from build123d import *

# Parameters (mm, degrees)
F0_R     = 25.4
F0_R_2   = 2.8345599267
F0_R_3   = 3.302
F1_DEPTH = 6.35
F2_DEPTH = 6.35
F3_R     = 4.0292814374
F4_DEPTH = 12.7


with BuildPart() as f1:
    # F0 (on Top) → F1 (new body)
    with BuildSketch(Plane.XY):
        Circle(F0_R)
        with Locations((-13.4316211013, -13.4316211013)):
            Circle(F0_R_2, mode=Mode.SUBTRACT)
        with Locations((0, -18.9951807261)):
            Circle(F0_R_2, mode=Mode.SUBTRACT)
        with Locations((-18.9951807261, 0)):
            Circle(F0_R_2, mode=Mode.SUBTRACT)
        Circle(F0_R_3, mode=Mode.SUBTRACT)
        with Locations((13.4316211013, -13.4316211013)):
            Circle(F0_R_2, mode=Mode.SUBTRACT)
        with Locations((18.9951807261, 0)):
            Circle(F0_R_2, mode=Mode.SUBTRACT)
        with Locations((-13.4316211013, 13.4316211013)):
            Circle(F0_R_2, mode=Mode.SUBTRACT)
        with Locations((0, 18.9951807261)):
            Circle(F0_R_2, mode=Mode.SUBTRACT)
        with Locations((13.4316211013, 13.4316211013)):
            Circle(F0_R_2, mode=Mode.SUBTRACT)
        with Locations((-18.9951807261, 0)):
            Circle(F0_R_2)
        with Locations((-13.4316211013, 13.4316211013)):
            Circle(F0_R_2)
        with Locations((0, 18.9951807261)):
            Circle(F0_R_2)
        with Locations((13.4316211013, 13.4316211013)):
            Circle(F0_R_2)
        with Locations((18.9951807261, 0)):
            Circle(F0_R_2)
        with Locations((0, -18.9951807261)):
            Circle(F0_R_2)
        with Locations((13.4316211013, -13.4316211013)):
            Circle(F0_R_2)
        with Locations((-13.4316211013, -13.4316211013)):
            Circle(F0_R_2)
    extrude(amount=F1_DEPTH)

    # F2 (add): a face of the model
    f2_faces = [f1.faces().sort_by_distance(p)[0] for p in [
        (-24.6815795103, 0, 6.35),
    ]]
    extrude(f2_faces, amount=F2_DEPTH)

    # F3 (on face) → F4 (join)
    with BuildSketch(Plane.XY.offset(12.7)):
        with Locations((0, 16.9805400074)):
            Circle(F3_R)
        with Locations((-14.7055790163, 8.4902700037)):
            Circle(F3_R)
        with Locations((-14.7055790163, -8.4902700037)):
            Circle(F3_R)
        with Locations((0, -16.9805400074)):
            Circle(F3_R)
        with Locations((14.7055790163, -8.4902700037)):
            Circle(F3_R)
        with Locations((14.7055790163, 8.4902700037)):
            Circle(F3_R)
    extrude(amount=F4_DEPTH)


solid = f1.part
CAD build for the part. Positions are in the model's coordinates, mm. A direction names the side the tool comes from. Give positions to 0.01 mm unless a question says otherwise; leave off trailing zeros. Write each loop counter-clockwise with the first axis right and the second up, starting at its lowest first coordinate (ties: lowest second). Pieces come first, ordered by that corner, then holes. Notation, with made-up numbers: (-39, -36.75) -> (7, -36.75) arc R19 cw to (7, -30.75) -> close; hole circle Ø9 at (-39.75, -39.5). An arc over 180 degrees is marked (long way). Return JSON: item names as keys, results as strings.
Item 1: Drill centre lines: probe 1 along Y at (x, z) = (0, 3.75); probe 2 along Z at (x, y) = (2.5, 6); probe 3 along Y at (x, z) = (-3, 19.75). Where is each one in solid material? Low to high.
Answer below:
{"probe 1": "y = -25.4 to -3.3, 3.3 to 25.4", "probe 2": "z = 0 to 12.7", "probe 3": "y = -19.67 to -14.29, 14.29 to 19.67"}
Item 2: Band-saw the part on D-D (x = 16). List the corners of the cut face in (y, z).
Answer below:
{"outline": "(-19.73, 0) -> (19.73, 0) -> (19.73, 12.7) -> (12.31, 12.7) -> (12.31, 25.4) -> (4.67, 25.4) -> (4.67, 12.7) -> (-4.67, 12.7) -> (-4.67, 25.4) -> (-12.31, 25.4) -> (-12.31, 12.7) -> (-19.73, 12.7) -> close"}
Item 3: Drop flat-ended pins along their axis: pin 1 (10 mm diameter, centred on x = 3.5, z = 18, fed in from +Y); pin 2 (1.5 mm diameter, centred on y = 19.5, z = 21.5, fed in from -X); pin 3 (1.5 mm diameter, centred on x = -12, z = 20, fed in from -Y); pin 4 (5.5 mm diameter, centred on x = 0, y = 0, fed in from +Z). Give the stop position or say it passes through.
Answer below:
{"pin 1": "stops at y = 21.01", "pin 2": "stops at x = -3.62", "pin 3": "stops at y = -12.01", "pin 4": "passes through"}
Item 4: Tool access for faces 1 (the cylindrical face through (10.68, 8.67, 18.96)), 2 (the flat face through (5, 0, 0)): list every direction of +Z, -Z, +X, -X, +Y, -Y with a clear straight run to the whole face (end or side of a thin tool).
Answer below:
{"face 1": "+Z", "face 2": "-Z, +X, -X, +Y, -Y"}
Item 5: Band-saw the part on B-B (x = 0). List the corners of the cut face in (y, z).
Answer below:
{"outline": "(-25.4, 0) -> (-3.3, 0) -> (-3.3, 12.7) -> (-12.95, 12.7) -> (-12.95, 25.4) -> (-21.01, 25.4) -> (-21.01, 12.7) -> (-25.4, 12.7) -> close; (3.3, 0) -> (25.4, 0) -> (25.4, 12.7) -> (21.01, 12.7) -> (21.01, 25.4) -> (12.95, 25.4) -> (12.95, 12.7) -> (3.3, 12.7) -> close"}
Item 6: Two-plate mould, pull along X, no slides. Class faces 3 (the flat face through (0, 17, 25.4)), 4 (the cylindrical face through (10.68, -8.31, 18.96)), 5 (the cylindrical face through (-0.525, 20.976, 18.961)): +X half, -X half, draft (parallel to the pull), parting line (faces both ways), or undercut.
Answer below:
{"face 3": "draft", "face 4": "undercut", "face 5": "parting line"}
Item 7: Band-saw the part on A-A (y = 0). List the corners of the cut face in (x, z).
Answer below:
{"outline": "(-25.4, 0) -> (-3.3, 0) -> (-3.3, 12.7) -> (-25.4, 12.7) -> close; (3.3, 0) -> (25.4, 0) -> (25.4, 12.7) -> (3.3, 12.7) -> close"}
Item 8: Band-saw the part on C-C (z = 5). List the corners of the cut face in (x, y).
Answer below:
{"outline": "circle Ø50.8 at (0, 0); hole circle Ø6.6 at (0, 0)"}
